```python
from build123d import *

# Parameters (mm, degrees)
F0_W     = 31.8
F0_H     = 15.8
F1_DEPTH = 9.6
F2_R     = 2.4
F3_DEPTH = 1.8
F4_R     = 1.3
F5_DEPTH = 8.7
F6_DEPTH = 8.5
F7_R     = 3.25685
F7_R_2   = 2.4
F8_DEPTH = 8.5


with BuildPart() as f1:
    # F0 (on Top) → F1 (new body)
    with BuildSketch(Plane.XY):
        Rectangle(F0_W, F0_H)
    extrude(amount=F1_DEPTH)

    # F2 (on face) → F3 (join)
    with BuildSketch(Plane.XY.offset(9.6)):
        with Locations((-12, 4)):
            Circle(F2_R)
        with Locations((-4, 4)):
            Circle(F2_R)
        with Locations((4, 4)):
            Circle(F2_R)
        with Locations((12, 4)):
            Circle(F2_R)
        with Locations((12, -4)):
            Circle(F2_R)
        with Locations((4, -4)):
            Circle(F2_R)
        with Locations((-4, -4)):
            Circle(F2_R)
        with Locations((-12, -4)):
            Circle(F2_R)
    extrude(amount=F3_DEPTH)

    # F4 (on face) → F5 (cut)
    with BuildSketch(Plane(origin=(0, 0, 0), x_dir=(1, 0, 0), z_dir=(0, 0, -1))):
        with Locations((-12, 4)):
            Circle(F4_R)
        with Locations((-4, 4)):
            Circle(F4_R)
        with Locations((4, 4)):
            Circle(F4_R)
        with Locations((12, 4)):
            Circle(F4_R)
        with Locations((12, -4)):
            Circle(F4_R)
        with Locations((4, -4)):
            Circle(F4_R)
        with Locations((-4, -4)):
            Circle(F4_R)
        with Locations((-12, -4)):
            Circle(F4_R)
    extrude(amount=-F5_DEPTH, mode=Mode.SUBTRACT)

    # F4 (on face) → F6 (cut)
    with BuildSketch(Plane(origin=(0, 0, 0), x_dir=(1, 0, 0), z_dir=(0, 0, -1))):
        Polygon((-12.3, 6.7), (-14.7, 6.7), (-14.7, 4.3), (-14.4, 4.3), (-14.4, 3.7), (-14.7, 3.7), (-14.7, -3.7), (-14.4, -3.7), (-14.4, -4.3), (-14.7, -4.3), (-14.7, -6.7), (-12.3, -6.7), (-12.3, -6.4), (-11.7, -6.4), (-11.7, -6.7), (-4.3, -6.7), (-4.3, -6.4), (-3.7, -6.4), (-3.7, -6.7), (3.7, -6.7), (3.7, -6.4), (4.3, -6.4), (4.3, -6.7), (11.7, -6.7), (11.7, -6.4), (12.3, -6.4), (12.3, -6.7), (14.7, -6.7), (14.7, -4.3), (14.4, -4.3), (14.4, -3.7), (14.7, -3.7), (14.7, 3.7), (14.4, 3.7), (14.4, 4.3), (14.7, 4.3), (14.7, 6.7), (12.3, 6.7), (12.3, 6.4), (11.7, 6.4), (11.7, 6.7), (4.3, 6.7), (4.3, 6.4), (3.7, 6.4), (3.7, 6.7), (-3.7, 6.7), (-3.7, 6.4), (-4.3, 6.4), (-4.3, 6.7), (-11.7, 6.7), (-11.7, 6.4), (-12.3, 6.4), align=None)
        with Locations((-12, -4)):
            Circle(F4_R, mode=Mode.SUBTRACT)
        with Locations((-4, -4)):
            Circle(F4_R, mode=Mode.SUBTRACT)
        with Locations((4, -4)):
            Circle(F4_R, mode=Mode.SUBTRACT)
        with Locations((12, -4)):
            Circle(F4_R, mode=Mode.SUBTRACT)
        with Locations((-12, 4)):
            Circle(F4_R, mode=Mode.SUBTRACT)
        with Locations((-4, 4)):
            Circle(F4_R, mode=Mode.SUBTRACT)
        with Locations((4, 4)):
            Circle(F4_R, mode=Mode.SUBTRACT)
        with Locations((12, 4)):
            Circle(F4_R, mode=Mode.SUBTRACT)
    extrude(amount=-F6_DEPTH, mode=Mode.SUBTRACT)

    # F7 (on face) → F8 (join, through all)
    with BuildSketch(Plane(origin=(0, 0, 8.5), x_dir=(1, 0, 0), z_dir=(0, 0, -1))):
        Circle(F7_R)
        Circle(F7_R_2, mode=Mode.SUBTRACT)
        with Locations((8, 0)):
            Circle(F7_R)
        with Locations((8, 0)):
            Circle(F7_R_2, mode=Mode.SUBTRACT)
        with Locations((-8, 0)):
            Circle(F7_R)
        with Locations((-8, 0)):
            Circle(F7_R_2, mode=Mode.SUBTRACT)
    extrude(amount=F8_DEPTH)


solid = f1.part
```
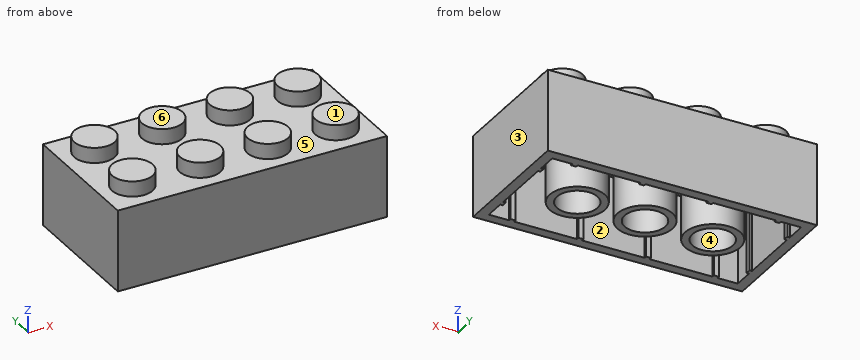
Can you work these out from the model? Positions are in its coordinate system, mm. Face numbers are marked on the shaded views. A direction names the side the tool comes from. Coordinates: 2 decimals unless noted, no trailing zeros. Loops run counter-clockwise (first coordinate to the right, second up) from the corner with the lowest first, then second, coordinate; pieces in that order, holes last. Notation, with made-up numbers: M -20,13.25 L 21,13.25 A19 ccw 21,44.25 Z; hole C 38.5,88.25 d6. An arc over 180 degrees is marked long. Put each result on its own line as item: value. Start each with the question number.
(1) We'd pull the mould along X, two halves only. Please class the marked faces 1, 2 and 3: +X half, -X half, draft (parallel to the pull), parting line (faces both ways), or undercut.
(2) Which directions (+Z, -Z, +X, -X, +Y, -Y) give clear straight access to the entire face, cutting with the end or side of a thin tool? Please do the marked faces 4, 5 and 6.
(3) I need wall thicknesses on probe 1 along X at (y, z) = (-4, 8.6); probe 2 along Y at (x, z) = (4, 8.6); probe 3 along Y at (x, z) = (8.5, 6). Which ranges of each line are inside material? Lowest first, please.
(4) Imagine slicing it at A-A on x = 12. List the corners of the cut face in (y, z) for me.
(5) Imagine slicing it at C-C on z = 5.5. Give the number of separate pieces and of enclosed holes in the cut face, and give its area (3 significant figures).
(6) Will these pins go through, and if not, where does the flat tip stop? pin 1 Ø2 at (x, y) = (-4, 4) entering from -Z; pin 2 Ø3 at (x, y) = (-12.5, 4.5) entering from -Z.
(7) Imagine slicing it at D-D on x = 0. List the corners of the cut face in (y, z) for me, and give its area (3 significant figures).
Worked answers:
1. face 1: draft
1. face 2: undercut
1. face 3: +X half
2. face 4: -Z
2. face 5: +Z
2. face 6: +Z, +X, -X, +Y, -Y
3. probe 1: x = -15.9 to -13.3, -10.7 to -5.3, -2.7 to 2.7, 5.3 to 10.7, 13.3 to 15.9
3. probe 2: y = -7.9 to -5.3, -2.7 to 2.7, 5.3 to 7.9
3. probe 3: y = -7.9 to -6.7, -3.22 to -2.35, 2.35 to 3.22, 6.7 to 7.9
4. outline: M -7.9,0 L -6.4,0 L -6.4,8.5 L -5.3,8.5 L -5.3,8.7 L -2.7,8.7 L -2.7,8.5 L 2.7,8.5 L 2.7,8.7 L 5.3,8.7 L 5.3,8.5 L 6.4,8.5 L 6.4,0 L 7.9,0 L 7.9,9.6 L 6.4,9.6 L 6.4,11.4 L 1.6,11.4 L 1.6,9.6 L -1.6,9.6 L -1.6,11.4 L -6.4,11.4 L -6.4,9.6 L -7.9,9.6 Z
5. separate pieces: 4
5. enclosed holes: 4
5. area: 156 mm2
6. pin 1: stops at z = 8.7
6. pin 2: stops at z = 8.5
7. outline: M -7.9,0 L -6.7,0 L -6.7,8.5 L -3.26,8.5 L -3.26,0 L -2.4,0 L -2.4,8.5 L 2.4,8.5 L 2.4,0 L 3.26,0 L 3.26,8.5 L 6.7,8.5 L 6.7,0 L 7.9,0 L 7.9,9.6 L -7.9,9.6 Z
7. area: 52.3 mm2
